CAD build for the part. Positions are in the model's coordinates, mm. Face numbers are marked on the shaded views. A direction names the side the tool comes from. Give positions to 0.01 mm unless a question says otherwise; leave off trailing zeros. Write each loop counter-clockwise with the first axis right and the second up, starting at its lowest first coordinate (ties: lowest second). Pieces come first, ordered by that corner, then holes. Notation, with made-up numbers: (-2, 25) -> (11, 25) arc R9 cw to (11, 42) -> close; hole circle Ø3 at (23.5, -32). An arc over 180 degrees is marked (long way). Answer as a JSON object with one key per item and string values.
```python
from build123d import *

# Parameters (mm, degrees)
F0_R     = 2.5
F1_DEPTH = 5


with BuildPart() as f1:
    # F0 (on Right) → F1 (new body)
    with BuildSketch(Plane.YZ):
        Polygon((-16.243222, 50), (-26.243222, 50), (-26.243222, 0), (33.756778, 0), (33.756778, 50), (23.756778, 50), (23.756778, 10), (-16.243222, 10), align=None)
        with Locations((-11.243222, 5)):
            Circle(F0_R, mode=Mode.SUBTRACT)
        with Locations((-21.243222, 20)):
            Circle(F0_R, mode=Mode.SUBTRACT)
        with Locations((18.756778, 5)):
            Circle(F0_R, mode=Mode.SUBTRACT)
        with Locations((28.756778, 20)):
            Circle(F0_R, mode=Mode.SUBTRACT)
        with Locations((-21.243222, 45)):
            Circle(F0_R, mode=Mode.SUBTRACT)
        with Locations((28.756778, 45)):
            Circle(F0_R, mode=Mode.SUBTRACT)
    extrude(amount=F1_DEPTH)


solid = f1.part
```
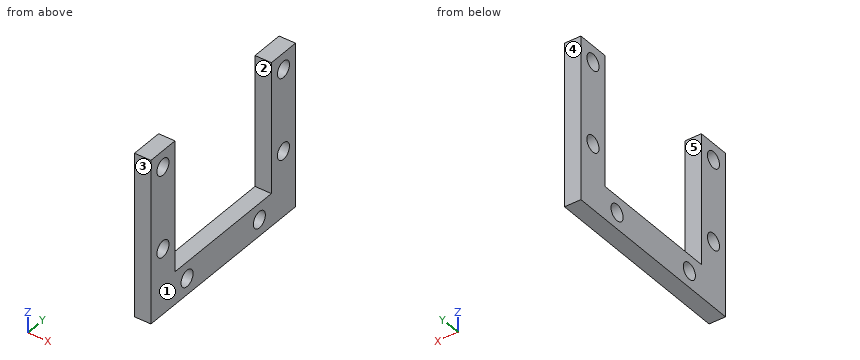
1) Slice it at C-C (x = 4.2). List the corners of the cut face in (y, z), then the cut area to 3 significant figures.
Model answer:
{"outline": "(-26.24, 0) -> (33.76, 0) -> (33.76, 50) -> (23.76, 50) -> (23.76, 10) -> (-16.24, 10) -> (-16.24, 50) -> (-26.24, 50) -> close; hole circle Ø5 at (-21.24, 20); hole circle Ø5 at (-21.24, 45); hole circle Ø5 at (-11.24, 5); hole circle Ø5 at (18.76, 5); hole circle Ø5 at (28.76, 20); hole circle Ø5 at (28.76, 45)", "area": "1,280 mm2"}
2) Pin check, flat tips, straight feed: pin 1 (3 mm diameter, centred on x = 4.5, y = 15, fed in from +Z); pin 2 (4 mm diameter, centred on y = 28.76, z = 20, fed in from -X). Stop position of each tip, or through.
Model answer:
{"pin 1": "stops at z = 10", "pin 2": "passes through"}
3) Slice it at B-B (z = 45). List the corners of the cut face in (x, y).
Model answer:
{"outline": "(0, -26.24) -> (5, -26.24) -> (5, -23.74) -> (0, -23.74) -> close; (0, -18.74) -> (5, -18.74) -> (5, -16.24) -> (0, -16.24) -> close; (0, 23.76) -> (5, 23.76) -> (5, 26.26) -> (0, 26.26) -> close; (0, 31.26) -> (5, 31.26) -> (5, 33.76) -> (0, 33.76) -> close"}
4) 3-axis set-ups, long thin cutter, end or side, ignore diameter. For the marked faces 4 and 5: which of +Z, -Z, +X, -X, +Y, -Y reach the whole face in a straight line?
Model answer:
{"face 4": "+Z, -Z, +X, -X, +Y", "face 5": "+Z, +X, -X"}
5) Slice it at D-D (y = 18.5). List the corners of the cut face in (x, z), then the cut area to 3 significant figures.
Model answer:
{"outline": "(0, 0) -> (5, 0) -> (5, 2.51) -> (0, 2.51) -> close; (0, 7.49) -> (5, 7.49) -> (5, 10) -> (0, 10) -> close", "area": "25.1 mm2"}
6) Wall check: probe 1 along Z at (x, y) = (4.25, -11); probe 2 along Y at (x, z) = (2.3, 41); probe 3 along Y at (x, z) = (4.2, 44.5). Give the ranges that are in metal, low to high.
Model answer:
{"probe 1": "z = 0 to 2.51, 7.49 to 10", "probe 2": "y = -26.24 to -16.24, 23.76 to 33.76", "probe 3": "y = -26.24 to -23.69, -18.79 to -16.24, 23.76 to 26.31, 31.21 to 33.76"}
7) Slice it at A-A (z = 5). List the corners of the cut face in (x, y).
Model answer:
{"outline": "(0, -26.24) -> (5, -26.24) -> (5, -13.74) -> (0, -13.74) -> close; (0, -8.74) -> (5, -8.74) -> (5, 16.26) -> (0, 16.26) -> close; (0, 21.26) -> (5, 21.26) -> (5, 33.76) -> (0, 33.76) -> close"}
8) Mould opens along Y. For the marked faces 1, 2 and 3 say: released by +Y, released by -Y, zero draft, split by the parting line, or undercut.
Model answer:
{"face 1": "zero draft", "face 2": "undercut", "face 3": "released by -Y"}
